Source: three-view drawing plus pictorial views. Frame: mm from the lowest corner of the part. A direction names the side the tool comes from. Coordinates: 2 decimals unless noted, no trailing zeros. Write each loop counter-clockwise with the first axis right and the second up, starting at its lowest first coordinate (ties: lowest second). Pieces come first, ordered by that corner, then holes. Notation, with made-up numbers: (20.5, 19) -> (59.5, 19) arc R17 ccw to (59.5, 23) -> close; hole circle Ø7 at (-15.75, 49). An arc over 180 degrees is marked (long way). Write item = value, one per line.
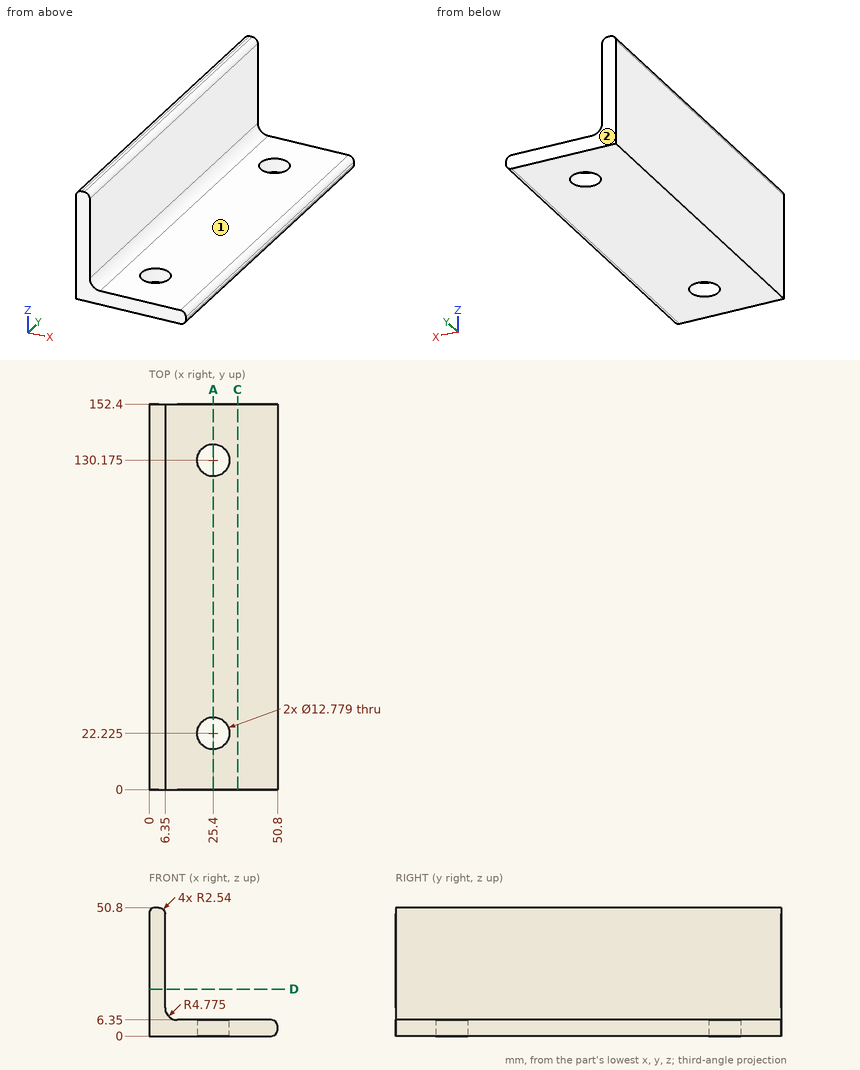
1) Cut plane C-C, the plane x = 35. Output: boundary loops of the cut face in (y, z).
Answer block:
outline = (0, 0) -> (152.4, 0) -> (152.4, 6.35) -> (0, 6.35) -> close
2) Material intervals for probe 1 along Y at (x, z) = (25.4, 1.5) (1 decimal); probe 2 along X at (y, z) = (146, 19.5), sorted ascending. Write a range as [from, to].
Answer block:
probe_1 = [0, 15.8], [28.6, 123.8], [136.6, 152.4]
probe_2 = [0, 6.35]
3) Cut plane D-D, the plane z = 18.5. Output: boundary loops of the cut face in (x, y).
Answer block:
outline = (0, 0) -> (6.35, 0) -> (6.35, 152.4) -> (0, 152.4) -> close
4) Cut plane A-A, the plane x = 25.4. Give the number of separate pieces and of enclosed holes in the cut face.
Answer block:
separate_pieces = 3
enclosed_holes = 0
5) First-contact query: pin 1 Ø5 at (x, y) = (15.5, 136.5) entering from -Z; pin 2 Ø6 at (y, z) = (71.5, 26.5) entering from +X; pin 3 Ø14.5 at (x, y) = (25.4, 22.225) entering from +Z; pin 4 Ø12 at (y, z) = (96.5, 14) entering from +X (1 decimal). Flat tips, straight axial feed; report the tip coordinate or a pass-through.
Answer block:
pin_1 = 0
pin_2 = 6.35
pin_3 = 6.35
pin_4 = 7.5
6) Reachability of the marked faces 1 and 2 from +Z, -Z, +X, -X, +Y, -Y: full face, straight path, thin tool, end or side. Return the list, or none.
Answer block:
face_1 = +Z, +X, +Y, -Y
face_2 = +Z, -Z, +X, -X, +Y
